from build123d import *

# Parameters (mm, degrees)
F0_W      = 20
F0_H      = 36
F1_DEPTH  = 12
F2_W      = 14
F2_H      = 24
F3_DEPTH  = 25
F4_R      = 3
F5_R      = 3
F6_W      = 34
F6_H      = 20
F7_DEPTH  = 6
F8_R      = 3
F9_R      = 3
F12_DEPTH = 6
F13_R     = 6
F14_DEPTH = 3
F15_R     = 6
F16_DEPTH = 3
F17_R     = 3
F18_DEPTH = 3
F19_R     = 3
F20_DEPTH = 3


with BuildPart() as f1:
    # F0 (on Top) → F1 (new body)
    with BuildSketch(Plane.XY):
        with Locations((-50.7072380185, 9.4144733921)):
            Rectangle(F0_W, F0_H)
    extrude(amount=F1_DEPTH)

    # F2 (on face) → F3 (cut)
    with BuildSketch(Plane.XY.offset(12)):
        with Locations((-53.7072380185, 9.3355261609)):
            Rectangle(F2_W, F2_H)
    extrude(amount=-F3_DEPTH, mode=Mode.SUBTRACT)

    # F4
    f4_edges = [f1.edges().sort_by_distance(p)[0] for p in [
        (-40.707238, -8.585527, 6),
    ]]
    fillet(f4_edges, radius=F4_R)

    # F5
    f5_edges = [f1.edges().sort_by_distance(p)[0] for p in [
        (-40.707238, 27.414473, 6),
        (-46.707238, -2.664474, 6),
        (-46.707238, 21.335526, 6),
    ]]
    fillet(f5_edges, radius=F5_R)

    # F6 (on Top) → F7 (join)
    with BuildSketch(Plane.XY):
        with Locations((-23.8486053348, 9.5559203671)):
            Rectangle(F6_W, F6_H)
    extrude(amount=F7_DEPTH)

    # F8
    f8_edges = [f1.edges().sort_by_distance(p)[0] for p in [
        (-40.707238, 19.55592, 3),
    ]]
    fillet(f8_edges, radius=F8_R)

    # F9
    f9_edges = [f1.edges().sort_by_distance(p)[0] for p in [
        (-40.707238, -0.44408, 3),
    ]]
    fillet(f9_edges, radius=F9_R)

    # F11 (on face) → F12 (join)
    with BuildSketch(Plane.XY.offset(6)):
        with BuildLine():
            ThreePointArc((-7.331625772, -0.4440796329), (0.0823230872, 2.2840744477), (3.2027962059, 9.5416298136))
            ThreePointArc((3.2027962059, 9.5416298136), (0.2556674153, 16.630847521), (-6.8486053348, 19.5414977068))
            Line((-6.8486053348, 19.5414977068), (-6.8486053348, 9.5559203671))
            Line((-6.8486053348, 9.5559203671), (-6.8486053348, -0.4440796329))
            Line((-6.8486053348, -0.4440796329), (-7.331625772, -0.4440796329))
        make_face()
    extrude(amount=-F12_DEPTH)

    # F13 (on face) → F14 (cut)
    with BuildSketch(Plane.XY.offset(6)):
        with Locations((-6.7972037941, 9.5416298136)):
            Circle(F13_R)
    extrude(amount=-F14_DEPTH, mode=Mode.SUBTRACT)

    # F15 (on face) → F16 (cut)
    with BuildSketch(Plane.XY.offset(6)):
        with Locations((-24.1282898933, 9.4736851752)):
            Circle(F15_R)
    extrude(amount=-F16_DEPTH, mode=Mode.SUBTRACT)

    # F17 (on face) → F18 (cut)
    with BuildSketch(Plane.XY.offset(3)):
        with Locations((-24.1282898933, 9.4736851752)):
            Circle(F17_R)
    extrude(amount=-F18_DEPTH, mode=Mode.SUBTRACT)

    # F19 (on face) → F20 (cut)
    with BuildSketch(Plane.XY.offset(3)):
        with Locations((-6.7972037941, 9.5416298136)):
            Circle(F19_R)
    extrude(amount=-F20_DEPTH, mode=Mode.SUBTRACT)


solid = f1.part
Design review of the part built by this model. Coordinates are the model's own, in mm. A direction names the side the tool comes from. Round coordinates to 2 decimals unless told otherwise and drop trailing zeros. Loops run counter-clockwise (first coordinate to the right, second up) from the corner with the lowest first, then second, coordinate; pieces in that order, holes last. Notation, with made-up numbers: M 85.5,-27 L 105.5,-27 A24 cw 105.5,3 Z; hole C 32.5,0.5 d4. An arc over 180 degrees is marked long. Answer as a JSON object with one key per item and string values.
Item 1: We need section C-C on x = -23. Give the boundary of the cut face in (y, z), and give its area (3 significant figures).
Answer sheet:
{"outline": "M -0.44,0 L 6.69,0 L 6.69,3 L 3.58,3 L 3.58,6 L -0.44,6 Z; M 12.25,0 L 19.56,0 L 19.56,6 L 15.37,6 L 15.37,3 L 12.25,3 Z", "area": "68.0 mm^2"}
Item 2: Machinability: for faces 5 (the flat face through (-52, -8.586, 6)), 6 (the flat face through (-22, 19.556, 3)), 7 (the flat face through (-55, -2.664, 6)), 8 (the cylindrical face through (-28.55, 13.53, 4.52)), which of the approach directions +Z, -Z, +X, -X, +Y, -Y give a long, thin tool a straight path to every point of the face, cutting with its end or side? Answer none if there is none.
Answer sheet:
{"face 5": "+Z, -Z, +X, -X, -Y", "face 6": "+Z, -Z, +X, +Y", "face 7": "+Z, -Z, -X", "face 8": "+Z"}
Item 3: We need section A-A on y = 8. Give the boundary of the cut face in (x, z), and give its area (3 significant figures).
Answer sheet:
{"outline": "M -46.71,0 L -26.74,0 L -26.74,3 L -29.94,3 L -29.94,6 L -40.71,6 L -40.71,12 L -46.71,12 Z; M -21.52,0 L -9.37,0 L -9.37,3 L -12.6,3 L -12.6,6 L -18.31,6 L -18.31,3 L -21.52,3 Z; M -4.22,0 L 3.08,0 L 3.08,6 L -1,6 L -1,3 L -4.22,3 Z", "area": "234 mm^2"}
Item 4: We need section B-B on z = 9. Give the boundary of the cut face in (x, y).
Answer sheet:
{"outline": "M -60.71,-8.59 L -43.71,-8.59 A3 ccw -40.71,-5.59 L -40.71,24.41 A3 ccw -43.71,27.41 L -60.71,27.41 L -60.71,21.34 L -49.71,21.34 A3 cw -46.71,18.34 L -46.71,0.34 A3 cw -49.71,-2.66 L -60.71,-2.66 Z"}
Item 5: Clearance check with flat-ended pins moving along their axes: P1, Ø9.5, axis at x = -6.8, y = 9.54, coming from the -Z side; P2, Ø3, axis at x = -28.5, z = 2.5, coming from the -Y side; P3, Ø6, axis at x = -14, z = 1.5, coming from the +Y side; P4, Ø13, axis at x = -24.5, y = 7, coming from the +Z side. State where each tip first meets the part, or that it passes through.
Answer sheet:
{"P1": "stops at z = 0", "P2": "stops at y = -0.44", "P3": "stops at y = 19.56", "P4": "stops at z = 6"}
Item 6: We need section D-D on z = 5. State how many separate pieces and enclosed holes the cut face has, and give its area (3 significant figures).
Answer sheet:
{"separate pieces": "1", "enclosed holes": "2", "area": "997 mm^2"}
Item 7: Wall thickness on L1, parallel to X at y = 9.5, z = 2; L2, parallel to Y at x = -52, z = 11; L3, parallel to X at y = 16.5, z = 11.75: over which ranges is each line inside the solid? List them lowest first. Write a range as from..to.
Answer sheet:
{"L1": "x = -46.71..-27.13, -21.13..-9.8, -3.8..3.2", "L2": "y = -8.59..-2.66, 21.34..27.41", "L3": "x = -46.71..-40.71"}
Item 8: The part is to be moulded in two halves that separate along X. For faces 1 (the flat face through (-46, 10, 12)), 2 (the flat face through (-27, 8, 3)), 3 (the flat face through (-10, 8, 3)), 4 (the cylindrical face through (-41.56, 26.51, 6.08)), say which applies: pulls with the +X half, pulls with the -X half, needs draft (parallel to the pull), parting line crosses it, or undercut.
Answer sheet:
{"face 1": "needs draft", "face 2": "undercut", "face 3": "undercut", "face 4": "pulls with the +X half"}
